Check sheet for the drawn part. Datum: minimum x, y, z corner. Units: mm. Give positions to 0.01 mm unless a question says otherwise; leave off trailing zeros. Loops run counter-clockwise (first coordinate to the right, second up) from the corner with the lowest first, then second, coordinate; pieces in that order, holes last.
1. Cross-section at D-D, the plane y = 3.5. State how many separate pieces and enclosed holes the cut face has, plus the area to 3 significant figures.
2. Cross-section at C-C, the plane z = 34. Record the cut outline in (x, y).
3. Release check for a two-part mould opening along X. For the marked faces 1, 2 and 3 record: +X half, -X half, draft (parallel to the pull), parting line (faces both ways), or undercut.
4. Go/stop test with a flat-tipped pin: pin 1 Ø4 at (y, z) = (2.5, 18) entering from +X. Record where the tip stops, or that it passes through.
5. Cross-section at B-B, the plane x = 28. Record the cut outline in (y, z).
6. Cross-section at A-A, the plane z = 28. Record the cut outline in (x, y).
7. Material ranges on L1, parallel to X at y = 5.25, z = 28; L2, parallel to Z at x = 26.5, y = 6.75; L3, parallel to X at y = 2, z = 22, recorded low to high.
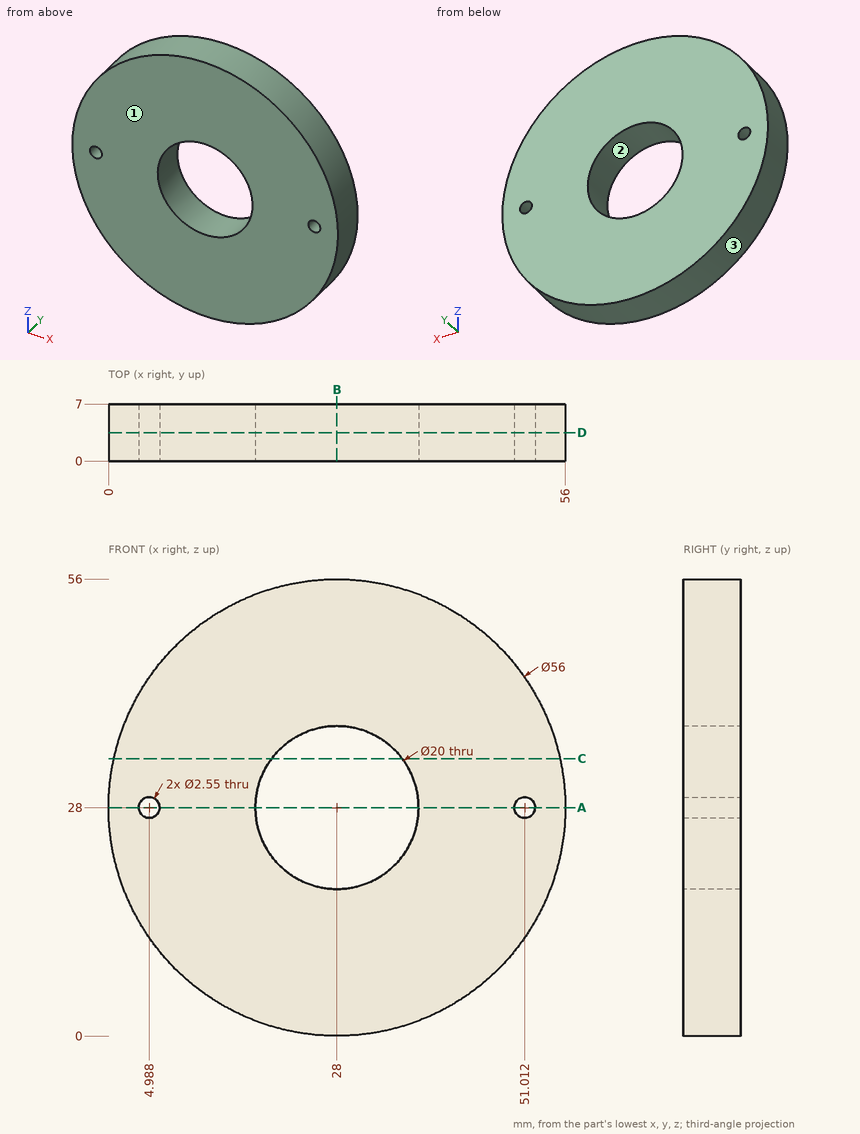
Result:
1. separate pieces: 1
1. enclosed holes: 3
1. area: 2,140 mm2
2. outline: (0.65, 0) - (20, 0) - (20, 7) - (0.65, 7) - close; (36, 0) - (55.35, 0) - (55.35, 7) - (36, 7) - close
3. face 1: draft
3. face 2: undercut
3. face 3: parting line
4. pin 1: stops at x = 54.83
5. outline: (0, 0) - (7, 0) - (7, 18) - (0, 18) - close; (0, 38) - (7, 38) - (7, 56) - (0, 56) - close
6. outline: (0, 0) - (3.71, 0) - (3.71, 7) - (0, 7) - close; (6.26, 0) - (18, 0) - (18, 7) - (6.26, 7) - close; (38, 0) - (49.74, 0) - (49.74, 7) - (38, 7) - close; (52.29, 0) - (56, 0) - (56, 7) - (52.29, 7) - close
7. L1: x = 0 to 3.71, 6.26 to 18, 38 to 49.74, 52.29 to 56
7. L2: z = 0.04 to 18.11, 37.89 to 55.96
7. L3: x = 0.65 to 20, 36 to 55.35
